Geometry: see drawing. Coordinates: mm, zero at the bounding-box minimum. Give positions to 0.01 mm unless a question says otherwise; leave off trailing zeros. Write each loop counter-clockwise with the first axis right and the second up, starting at its lowest first coordinate (ties: lowest second). Pieces come first, ordered by that corner, then holes. Notation, with made-up numbers: (81, 89) -> (95, 89) arc R29 cw to (95, 110) -> close; hole circle Ø1 at (-35, 55). An arc over 180 degrees is marked (long way). Answer as a JSON object with one key per item and string values. Group by question number.
Item 1: Section query B-B on x = 7. Return the cut outline in (y, z).
Item 2: First-contact query: pin 1 Ø0.8 at (y, z) = (35, 3) entering from +X. Flat tip, straight axial feed; report the tip coordinate or a pass-through.
Item 3: Ray query, probe 1 along Y at (x, z) = (7, 2.55); probe 2 along Y at (x, z) = (8.5, 2.65); probe 3 along X at (y, z) = (22, 4.75). Return the intervals inside material, ascending. Write a range as from..to.
Item 4: Section query A-A on y = 52.5. Return the cut outline in (x, z).
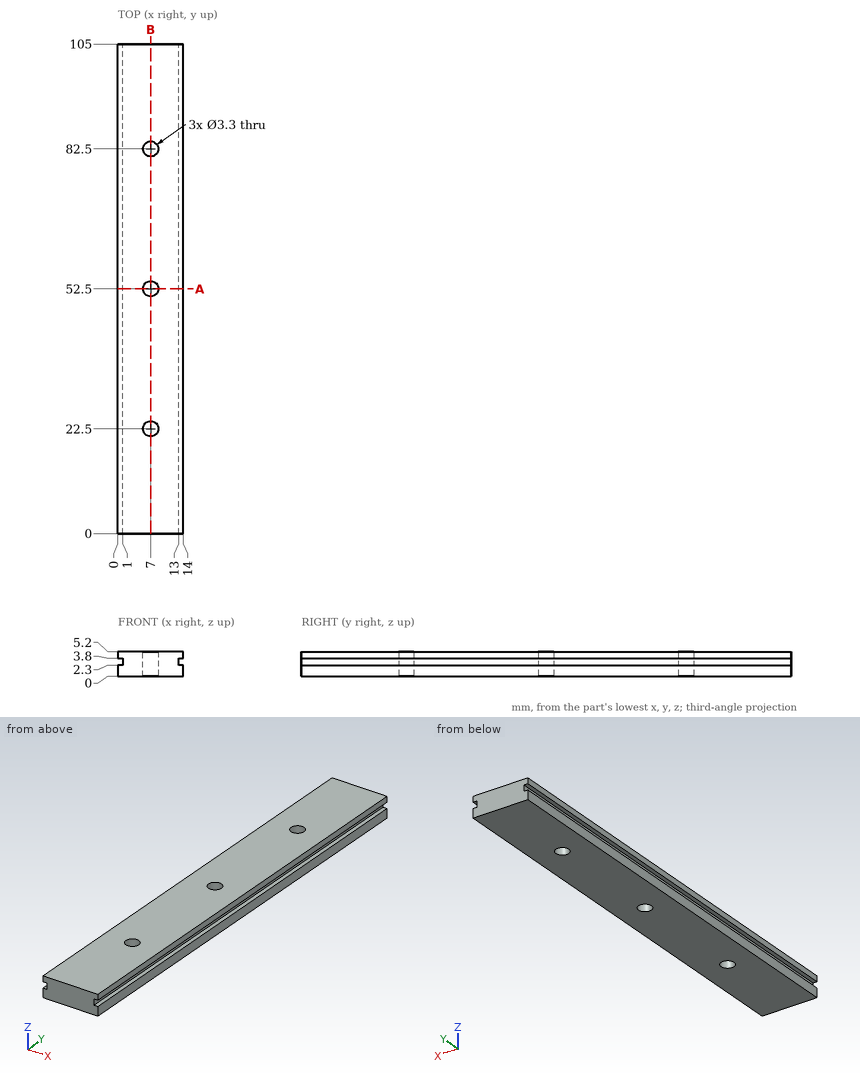
Worked answers:
{
 "1": {"outline": "(0, 0) -> (20.85, 0) -> (20.85, 5.2) -> (0, 5.2) -> close; (24.15, 0) -> (50.85, 0) -> (50.85, 5.2) -> (24.15, 5.2) -> close; (54.15, 0) -> (80.85, 0) -> (80.85, 5.2) -> (54.15, 5.2) -> close; (84.15, 0) -> (105, 0) -> (105, 5.2) -> (84.15, 5.2) -> close"},
 "2": {"pin 1": "x = 13"},
 "3": {"probe 1": "0..20.85, 24.15..50.85, 54.15..80.85, 84.15..105", "probe 2": "0..21.81, 23.19..51.81, 53.19..81.81, 83.19..105", "probe 3": "0..5.43, 8.57..14"},
 "4": {"outline": "(0, 0) -> (5.35, 0) -> (5.35, 5.2) -> (0, 5.2) -> (0, 3.8) -> (1, 3.8) -> (1, 2.3) -> (0, 2.3) -> close; (8.65, 0) -> (14, 0) -> (14, 2.3) -> (13, 2.3) -> (13, 3.8) -> (14, 3.8) -> (14, 5.2) -> (8.65, 5.2) -> close"}
}
